Model file for the job. Use its own axes, mm. Face numbers are marked on the shaded views. A direction names the side the tool comes from. Give positions to 0.01 mm unless a question says otherwise; leave off trailing zeros. Loops run counter-clockwise (first coordinate to the right, second up) from the corner with the lowest first, then second, coordinate; pieces in that order, holes last. Notation, with made-up numbers: (5.5, 37.25) - (49.5, 37.25) arc R21 cw to (49.5, 75.25) - close; hole circle Ø6 at (13, 12). An arc over 180 degrees is marked (long way). Use a Markdown table: item, result.
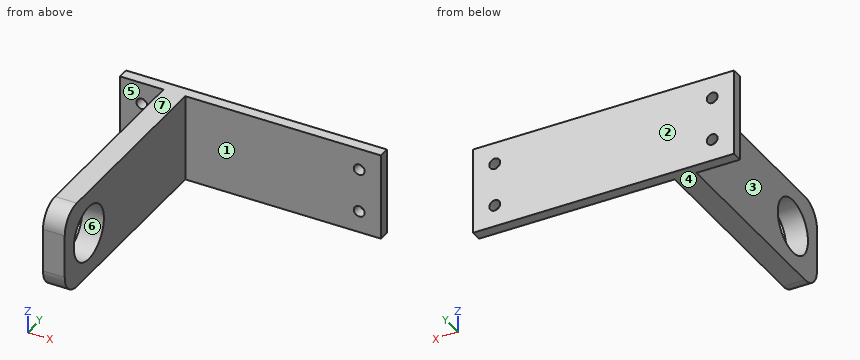
from build123d import *

# Parameters (mm, degrees)
F0_W     = 152.4
F0_H     = 50.8
F1_DEPTH = 6.35
F3_D     = 6.35
F4_W     = 12.7
F4_H     = 50.8
F5_DEPTH = 127
F6_R     = 12.7
F8_D     = 31.75


with BuildPart() as f1:
    # F0 (on Front) → F1 (new body)
    with BuildSketch(Plane.XZ):
        with Locations((76.2, 25.4)):
            Rectangle(F0_W, F0_H)
    extrude(amount=F1_DEPTH)

    # F3 (through all)
    with Locations(Plane.XZ.offset(6.35)):
        with Locations((12.7, 38.1), (12.7, 12.7), (139.7, 38.1), (139.7, 12.7)):
            Hole(F3_D / 2)

    # F4 (on face) → F5 (join)
    with BuildSketch(Plane.XZ.offset(6.35)):
        with Locations((31.75, 25.4)):
            Rectangle(F4_W, F4_H)
    extrude(amount=F5_DEPTH)

    # F6
    f6_edges = [f1.edges().sort_by_distance(p)[0] for p in [
        (31.75, -133.35, 0),
        (31.75, -133.35, 50.8),
    ]]
    fillet(f6_edges, radius=F6_R)

    # F8 (through all)
    with Locations(Plane.YZ.offset(38.1)):
        with Locations((-107.95, 25.4)):
            Hole(F8_D / 2)


solid = f1.part
(1) Slice it at B-B, the plane z = 25.4. Write the cut outline in (x, y) (3 decimals).
Computed:
| item | result |
|---|---|
| outline | (0, -6.35) - (25.4, -6.35) - (25.4, -92.075) - (38.1, -92.075) - (38.1, -6.35) - (152.4, -6.35) - (152.4, 0) - (0, 0) - close; (25.4, -133.35) - (38.1, -133.35) - (38.1, -123.825) - (25.4, -123.825) - close |
(2) Slice it at A-A, the plane y = -107.95. Write the cut outline in (x, z) (3 decimals), plus the area to 3 significant figures.
Computed:
| item | result |
|---|---|
| outline | (25.4, 0) - (38.1, 0) - (38.1, 9.525) - (25.4, 9.525) - close; (25.4, 41.275) - (38.1, 41.275) - (38.1, 50.8) - (25.4, 50.8) - close |
| area | 242 mm² |
(3) Drill centre lines: probe 1 along Z at (x, y) = (139.7, -3.5) (3 decimals); probe 2 along X at (y, z) = (-4, 38); probe 3 along Y at (x, z) = (28, 25). Where is each one in solid material? Low to high. Write a range as [from, to].
Computed:
| item | result |
|---|---|
| probe 1 | [0, 9.525], [15.875, 34.925], [41.275, 50.8] |
| probe 2 | [0, 9.53], [15.87, 136.53], [142.87, 152.4] |
| probe 3 | [-133.35, -123.82], [-92.08, 0] |
(4) Mould opens along Z. For the marked faces 4, 5, 6 and 7 say: pulls with the +Z half, pulls with the -Z half, needs draft (parallel to the pull), parting line crosses it, or undercut.
Computed:
| item | result |
|---|---|
| face 4 | pulls with the -Z half |
| face 5 | needs draft |
| face 6 | undercut |
| face 7 | pulls with the +Z half |
(5) Slice it at D-D, the plane x = 32. Write the cut outline in (y, z) (3 decimals).
Computed:
| item | result |
|---|---|
| outline | (-133.35, 12.7) arc R12.7 ccw to (-120.65, 0) - (0, 0) - (0, 50.8) - (-120.65, 50.8) arc R12.7 ccw to (-133.35, 38.1) - close; hole circle Ø31.75 at (-107.95, 25.4) |
(6) Slice it at C-C, the plane x = 12.7. Write the cut outline in (y, z) (3 decimals), plus the area to 3 significant figures.
Computed:
| item | result |
|---|---|
| outline | (-6.35, 0) - (0, 0) - (0, 9.525) - (-6.35, 9.525) - close; (-6.35, 15.875) - (0, 15.875) - (0, 34.925) - (-6.35, 34.925) - close; (-6.35, 41.275) - (0, 41.275) - (0, 50.8) - (-6.35, 50.8) - close |
| area | 242 mm² |
(7) 3-axis set-ups, long thin cutter, end or side, ignore diameter. For the marked faces 1, 2 and 3: which of +Z, -Z, +X, -X, +Y, -Y reach the whole face in a straight line?
Computed:
| item | result |
|---|---|
| face 1 | +Z, -Z, +X, -Y |
| face 2 | +Z, -Z, +X, -X, +Y |
| face 3 | +Z, -Z, -X, -Y |
(8) Pin check, flat tips, straight feed: P1, Ø5, axis at x = 12.7, z = 12.7, coming from the -Y side; P2, Ø15, axis at y = -50.5, z = 24, coming from the +X side; P3, Ø20.5, axis at x = 11, z = 21, coming from the -Y side; P4, Ø2, axis at y = -79.5, z = 45.5, coming from the -X side. Stop position of each tip, or through.
Computed:
| item | result |
|---|---|
| P1 | through |
| P2 | x = 38.1 |
| P3 | y = -6.35 |
| P4 | x = 25.4 |
